from build123d import *

# Parameters (mm, degrees)
F0_R     = 11.45
F1_DEPTH = 7.62


# Not quite as in the source:
# - a feature names something its author has since deleted; it is built from what else it names


with BuildPart() as f1:
    # F0 (on Top) → F1 (new body)
    with BuildSketch(Plane.XY):
        with BuildLine():
            ThreePointArc((-10.038027058, 16.1907539288), (0, 19.05), (10.038027058, 16.1907539288))
            ThreePointArc((10.038027058, 16.1907539288), (8.1892299167, 26.451450684), (10.618228457, 36.59047997))
            ThreePointArc((10.618228457, 36.59047997), (0, 38.1), (-10.618228457, 36.59047997))
            ThreePointArc((-10.618228457, 36.59047997), (-8.1892299167, 26.451450684), (-10.038027058, 16.1907539288))
        make_face()
        with BuildLine():
            ThreePointArc((16.1907539288, -10.038027058), (18.3212494435, -5.2186510544), (19.05, 0))
            ThreePointArc((19.05, 0), (18.3212494435, 5.2186510544), (16.1907539288, 10.038027058))
            ThreePointArc((16.1907539288, 10.038027058), (15.2571196867, 11.4071380664), (14.208032523, 12.6899295438))
            ThreePointArc((14.208032523, 12.6899295438), (13.3304286547, 13.6089004655), (12.3935124609, 14.4673200311))
            ThreePointArc((12.3935124609, 14.4673200311), (11.2488242673, 15.3742138857), (10.038027058, 16.1907539288))
            ThreePointArc((10.038027058, 16.1907539288), (0, 19.05), (-10.038027058, 16.1907539288))
            ThreePointArc((-10.038027058, 16.1907539288), (-11.4071380664, 15.2571196867), (-12.6899295437, 14.208032523))
            ThreePointArc((-12.6899295437, 14.208032523), (-13.6089004655, 13.3304286548), (-14.467320031, 12.3935124609))
            ThreePointArc((-14.467320031, 12.3935124609), (-15.3742138857, 11.2488242673), (-16.1907539288, 10.038027058))
            ThreePointArc((-16.1907539288, 10.038027058), (-19.05, 0), (-16.1907539288, -10.038027058))
            ThreePointArc((-16.1907539288, -10.038027058), (-15.2571196867, -11.4071380664), (-14.208032523, -12.6899295437))
            ThreePointArc((-14.208032523, -12.6899295437), (-13.3304286548, -13.6089004655), (-12.3935124609, -14.467320031))
            ThreePointArc((-12.3935124609, -14.467320031), (-11.2488242673, -15.3742138857), (-10.038027058, -16.1907539288))
            ThreePointArc((-10.038027058, -16.1907539288), (0, -19.05), (10.038027058, -16.1907539288))
            ThreePointArc((10.038027058, -16.1907539288), (11.4071380664, -15.2571196867), (12.6899295438, -14.208032523))
            ThreePointArc((12.6899295438, -14.208032523), (13.6089004655, -13.3304286547), (14.4673200311, -12.3935124609))
            ThreePointArc((14.4673200311, -12.3935124609), (15.3742138857, -11.2488242673), (16.1907539288, -10.038027058))
        make_face()
        Circle(F0_R, mode=Mode.SUBTRACT)
        with BuildLine():
            ThreePointArc((-10.618228457, 36.59047997), (0, 38.1), (10.618228457, 36.59047997))
            ThreePointArc((10.618228457, 36.59047997), (10.9631553547, 37.2915593412), (11.3294826074, 37.9816978733))
            ThreePointArc((11.3294826074, 37.9816978733), (9.6714472488, 40.5242467677), (7.4026469551, 42.5407242305))
            ThreePointArc((7.4026469551, 42.5407242305), (0, 43.18), (-7.4026469551, 42.5407242305))
            ThreePointArc((-7.4026469551, 42.5407242305), (-9.6714472488, 40.5242467677), (-11.3294826074, 37.9816978733))
            ThreePointArc((-11.3294826074, 37.9816978733), (-10.9631553547, 37.2915593412), (-10.618228457, 36.59047997))
        make_face()
        with BuildLine():
            ThreePointArc((-27.6564265836, 26.2055732359), (-19.8292429656, 32.5332310632), (-10.618228457, 36.59047997))
            ThreePointArc((-10.618228457, 36.59047997), (-10.9631553547, 37.2915593412), (-11.3294826074, 37.9816978733))
            ThreePointArc((-11.3294826074, 37.9816978733), (-9.6714472488, 40.5242467677), (-7.4026469551, 42.5407242305))
            ThreePointArc((-7.4026469551, 42.5407242305), (-30.5262465043, 30.5394936821), (-42.5375084691, 7.4211032363))
            ThreePointArc((-42.5375084691, 7.4211032363), (-42.4698240182, 7.5132687267), (-42.401220917, 7.6047524795))
            ThreePointArc((-42.401220917, 7.6047524795), (-40.430781391, 9.7510814924), (-37.9816978733, 11.3294826074))
            ThreePointArc((-37.9816978733, 11.3294826074), (-37.2915593412, 10.9631553547), (-36.59047997, 10.618228457))
            ThreePointArc((-36.59047997, 10.618228457), (-33.6685368778, 17.8336654815), (-29.3410352271, 24.3046014533))
            ThreePointArc((-29.3410352271, 24.3046014533), (-28.5145767397, 25.2691296517), (-27.6564265836, 26.2055732359))
        make_face()
        with BuildLine():
            ThreePointArc((-11.3294826074, -37.9816978733), (-10.9631553547, -37.2915593412), (-10.618228457, -36.59047997))
            ThreePointArc((-10.618228457, -36.59047997), (-17.8336654815, -33.6685368778), (-24.3046014533, -29.3410352271))
            ThreePointArc((-24.3046014533, -29.3410352271), (-25.2691296517, -28.5145767397), (-26.2055732359, -27.6564265836))
            ThreePointArc((-26.2055732359, -27.6564265836), (-32.5332310632, -19.8292429656), (-36.59047997, -10.618228457))
            ThreePointArc((-36.59047997, -10.618228457), (-37.2915593412, -10.9631553547), (-37.9816978733, -11.3294826074))
            ThreePointArc((-37.9816978733, -11.3294826074), (-40.5242467677, -9.6714472488), (-42.5407242305, -7.4026469551))
            ThreePointArc((-42.5407242305, -7.4026469551), (-30.5328708116, -30.5328708116), (-7.4026469551, -42.5407242305))
            ThreePointArc((-7.4026469551, -42.5407242305), (-9.6714472488, -40.5242467677), (-11.3294826074, -37.9816978733))
        make_face()
        with BuildLine():
            Line((-24.3046014533, -29.3410352271), (-12.3935124609, -14.467320031))
            ThreePointArc((-12.3935124609, -14.467320031), (-13.3304286548, -13.6089004655), (-14.208032523, -12.6899295437))
            Line((-14.208032523, -12.6899295437), (-26.2055732359, -27.6564265836))
            ThreePointArc((-26.2055732359, -27.6564265836), (-25.2691296517, -28.5145767397), (-24.3046014533, -29.3410352271))
        make_face()
        with BuildLine():
            ThreePointArc((10.6182284569, -36.59047997), (8.1892299167, -26.451450684), (10.038027058, -16.1907539288))
            ThreePointArc((10.038027058, -16.1907539288), (0, -19.05), (-10.038027058, -16.1907539288))
            ThreePointArc((-10.038027058, -16.1907539288), (-8.1892299167, -26.451450684), (-10.618228457, -36.59047997))
            ThreePointArc((-10.618228457, -36.59047997), (0, -38.1), (10.6182284569, -36.59047997))
        make_face()
        with BuildLine():
            ThreePointArc((11.3294826074, -37.9816978733), (10.9631553547, -37.2915593412), (10.6182284569, -36.59047997))
            ThreePointArc((10.6182284569, -36.59047997), (0, -38.1), (-10.618228457, -36.59047997))
            ThreePointArc((-10.618228457, -36.59047997), (-10.9631553547, -37.2915593412), (-11.3294826074, -37.9816978733))
            ThreePointArc((-11.3294826074, -37.9816978733), (-9.6714472488, -40.5242467677), (-7.4026469551, -42.5407242305))
            ThreePointArc((-7.4026469551, -42.5407242305), (0, -43.18), (7.4026469551, -42.5407242305))
            ThreePointArc((7.4026469551, -42.5407242305), (9.6714472488, -40.5242467677), (11.3294826074, -37.9816978733))
        make_face()
        with BuildLine():
            ThreePointArc((37.9816978733, 11.3294826074), (37.2915593412, 10.9631553547), (36.59047997, 10.6182284569))
            ThreePointArc((36.59047997, 10.6182284569), (37.7207322759, 5.3624953679), (38.1, 0))
            ThreePointArc((38.1, 0), (37.7207322759, -5.3624953679), (36.59047997, -10.618228457))
            ThreePointArc((36.59047997, -10.618228457), (37.2915593412, -10.9631553547), (37.9816978733, -11.3294826074))
            ThreePointArc((37.9816978733, -11.3294826074), (40.5242467677, -9.6714472488), (42.5407242305, -7.4026469551))
            ThreePointArc((42.5407242305, -7.4026469551), (43.0198841948, -3.7150994419), (43.18, 0))
            ThreePointArc((43.18, 0), (43.0198841948, 3.7150994419), (42.5407242305, 7.4026469551))
            ThreePointArc((42.5407242305, 7.4026469551), (40.5242467677, 9.6714472488), (37.9816978733, 11.3294826074))
        make_face()
        with BuildLine():
            ThreePointArc((16.1907539288, 10.038027058), (18.3212494435, 5.2186510544), (19.05, 0))
            ThreePointArc((19.05, 0), (18.3212494435, -5.2186510544), (16.1907539288, -10.038027058))
            ThreePointArc((16.1907539288, -10.038027058), (26.451450684, -8.1892299167), (36.59047997, -10.618228457))
            ThreePointArc((36.59047997, -10.618228457), (37.7207322759, -5.3624953679), (38.1, 0))
            ThreePointArc((38.1, 0), (37.7207322759, 5.3624953679), (36.59047997, 10.6182284569))
            ThreePointArc((36.59047997, 10.6182284569), (26.451450684, 8.1892299167), (16.1907539288, 10.038027058))
        make_face()
        with BuildLine():
            Line((29.3410352271, -24.3046014533), (14.467320031, -12.3935124609))
            ThreePointArc((14.4673200311, -12.3935124609), (13.6089004655, -13.3304286547), (12.6899295438, -14.208032523))
            Line((12.6899295437, -14.208032523), (27.6564265836, -26.2055732359))
            ThreePointArc((27.6564265836, -26.2055732359), (28.5145767397, -25.2691296517), (29.3410352271, -24.3046014533))
        make_face()
        with BuildLine():
            ThreePointArc((-14.467320031, 12.3935124609), (-13.6089004655, 13.3304286548), (-12.6899295437, 14.208032523))
            Line((-12.6899295437, 14.208032523), (-27.6564265836, 26.2055732359))
            ThreePointArc((-27.6564265836, 26.2055732359), (-28.5145767397, 25.2691296517), (-29.3410352271, 24.3046014533))
            Line((-29.3410352271, 24.3046014533), (-14.467320031, 12.3935124609))
        make_face()
        with BuildLine():
            ThreePointArc((12.3935124609, 14.4673200311), (13.3304286547, 13.6089004655), (14.208032523, 12.6899295438))
            Line((14.208032523, 12.6899295438), (26.2055732359, 27.6564265836))
            ThreePointArc((26.2055732359, 27.6564265836), (25.2691296517, 28.5145767397), (24.3046014533, 29.3410352271))
            Line((24.3046014533, 29.3410352271), (12.3935124609, 14.4673200311))
        make_face()
        with BuildLine():
            ThreePointArc((37.9816978733, -11.3294826074), (37.2915593412, -10.9631553547), (36.59047997, -10.618228457))
            ThreePointArc((36.59047997, -10.618228457), (33.6685368778, -17.8336654815), (29.3410352271, -24.3046014533))
            ThreePointArc((29.3410352271, -24.3046014533), (28.5145767397, -25.2691296517), (27.6564265836, -26.2055732359))
            ThreePointArc((27.6564265836, -26.2055732359), (19.8292429656, -32.5332310632), (10.6182284569, -36.59047997))
            ThreePointArc((10.6182284569, -36.59047997), (10.9631553547, -37.2915593412), (11.3294826074, -37.9816978733))
            ThreePointArc((11.3294826074, -37.9816978733), (9.6714472488, -40.5242467677), (7.4026469551, -42.5407242305))
            ThreePointArc((7.4026469551, -42.5407242305), (30.5328708116, -30.5328708116), (42.5407242305, -7.4026469551))
            ThreePointArc((42.5407242305, -7.4026469551), (40.5242467677, -9.6714472488), (37.9816978733, -11.3294826074))
        make_face()
        with BuildLine():
            ThreePointArc((26.2055732359, 27.6564265836), (32.5332310632, 19.8292429656), (36.59047997, 10.6182284569))
            ThreePointArc((36.59047997, 10.6182284569), (37.2915593412, 10.9631553547), (37.9816978733, 11.3294826074))
            ThreePointArc((37.9816978733, 11.3294826074), (40.5242467677, 9.6714472488), (42.5407242305, 7.4026469551))
            ThreePointArc((42.5407242305, 7.4026469551), (30.5328708116, 30.5328708116), (7.4026469551, 42.5407242305))
            ThreePointArc((7.4026469551, 42.5407242305), (9.6714472488, 40.5242467677), (11.3294826074, 37.9816978733))
            ThreePointArc((11.3294826074, 37.9816978733), (10.9631553547, 37.2915593412), (10.618228457, 36.59047997))
            ThreePointArc((10.618228457, 36.59047997), (17.8336654815, 33.6685368778), (24.3046014533, 29.3410352271))
            ThreePointArc((24.3046014533, 29.3410352271), (25.2691296517, 28.5145767397), (26.2055732359, 27.6564265836))
        make_face()
        with BuildLine():
            ThreePointArc((-16.1907539288, -10.038027058), (-19.05, 0), (-16.1907539288, 10.038027058))
            ThreePointArc((-16.1907539288, 10.038027058), (-26.451450684, 8.1892299167), (-36.59047997, 10.618228457))
            ThreePointArc((-36.59047997, 10.618228457), (-38.1, 0), (-36.59047997, -10.618228457))
            ThreePointArc((-36.59047997, -10.618228457), (-26.451450684, -8.1892299167), (-16.1907539288, -10.038027058))
        make_face()
        with BuildLine():
            ThreePointArc((-42.5407242305, 7.4026469551), (-43.18, 0), (-42.5407242305, -7.4026469551))
            ThreePointArc((-42.5407242305, -7.4026469551), (-40.5242467677, -9.6714472488), (-37.9816978733, -11.3294826074))
            ThreePointArc((-37.9816978733, -11.3294826074), (-37.2915593412, -10.9631553547), (-36.59047997, -10.618228457))
            ThreePointArc((-36.59047997, -10.618228457), (-38.1, 0), (-36.59047997, 10.618228457))
            ThreePointArc((-36.59047997, 10.618228457), (-37.2915593412, 10.9631553547), (-37.9816978733, 11.3294826074))
            ThreePointArc((-37.9816978733, 11.3294826074), (-40.430781391, 9.7510814924), (-42.401220917, 7.6047524795))
            ThreePointArc((-42.401220917, 7.6047524795), (-42.4715153756, 7.5040743862), (-42.5407242305, 7.4026469551))
        make_face()
    extrude(amount=F1_DEPTH)


solid = f1.part
The listing builds one solid part. Answer for the finished solid, in the listing's coordinates (mm). A direction names the side the tool comes from. Coordinates: 2 decimals unless noted, no trailing zeros. Order: outer loops, then holes, each group sorted by start corner. A loop starts at its lowest first (then second) coordinate and runs counter-clockwise, first axis right, second up. Notation, with made-up numbers: (64.5, 42) -> (84.5, 42) arc R25 ccw to (84.5, 64) -> close; hole circle Ø6 at (-7, 27). An arc over 180 degrees is marked (long way). Answer in a Markdown table with one row per item. Add a question column.
Item 1: Determine the mould class of faces 3 (the face through (-26.598, -8.194, 3.757)), 4 (the face through (9, -9, 0)), 5 (the face through (19.95, -32.46, 3.76)) for opening direction Y: +Y half, -Y half, draft (parallel to the pull), parting line (faces both ways), or undercut.
Item 2: Find the intervals of material crossed by L1, parallel to Y at x = -22, z = 3.75; L2, parallel to X at y = -24, z = 3.5; L3, parallel to Y at x = -23, z = 2.5, in increasing order. Write a range as from..to.
Item 3: Find section B-B (y = 33). Write down the section's boundary in (x, z).
Item 4: Each of these flat-tipped pins is pushed along its axis until it touches: P1, Ø1.5, axis at y = 33.5, z = 4.5, coming from the -X side; P2, Ø1.5, axis at x = 20, y = 5, coming from the -Z side; P3, Ø18.5, axis at x = 0, y = 0, coming from the +Z side; P4, Ø1.5, axis at y = -26, z = 2.5, coming from the +X side. Where does it stop, or does it pass through?
Item 5: Find section C-C (x = 17.5). Write down the section's boundary in (y, z), then the cut area to 3 significant figures.
Item 6: Find section A-A (x = 0). Write down the section's boundary in (y, z).
Item 7: Which of the six approach directions +Z, -Z, +X, -X, +Y, -Y give full straight-line access (tool end or side, diameter ignored) to faces 1 (the face through (33.72, -17.74, 3.76)), 2 (the face through (9, -9, 7.62))?
Item 8: Find section D-D (x = 32). Write down the section's boundary in (y, z).
Result set:
| question | item | result |
|---|---|---|
| 1 | face 3 | undercut |
| 1 | face 4 | draft |
| 1 | face 5 | undercut |
| 2 | L1 | y = -37.16..-31.11, -26.46..-22.41, -8.45..8.45, 18.43..21.67, 31.11..37.16 |
| 2 | L2 | x = -35.9..-29.59, -23.27..-20.03, -8.24..8.24, 24.91..28.96, 29.59..35.9 |
| 2 | L3 | y = -36.54..-30.37, -27.71..-23.66, -8.33..8.33, 19.23..22.47, 30.37..36.54 |
| 3 | outline | (-27.85, 0) -> (-19.04, 0) -> (-19.04, 7.62) -> (-27.85, 7.62) -> close; (-9.24, 0) -> (9.24, 0) -> (9.24, 7.62) -> (-9.24, 7.62) -> close; (19.04, 0) -> (27.85, 0) -> (27.85, 7.62) -> (19.04, 7.62) -> close |
| 4 | P1 | stops at x = -28.14 |
| 4 | P2 | stops at z = 0 |
| 4 | P3 | passes through |
| 4 | P4 | stops at x = 35.03 |
| 5 | outline | (-39.47, 0) -> (-33.84, 0) -> (-33.84, 7.62) -> (-39.47, 7.62) -> close; (-18.06, 0) -> (-14.82, 0) -> (-14.82, 7.62) -> (-18.06, 7.62) -> close; (-9.55, 0) -> (9.55, 0) -> (9.55, 7.62) -> (-9.55, 7.62) -> close; (16.8, 0) -> (20.84, 0) -> (20.84, 7.62) -> (16.8, 7.62) -> close; (33.84, 0) -> (39.47, 0) -> (39.47, 7.62) -> (33.84, 7.62) -> close |
| 5 | area | 287 mm² |
| 6 | outline | (-43.18, 0) -> (-11.45, 0) -> (-11.45, 7.62) -> (-43.18, 7.62) -> close; (11.45, 0) -> (43.18, 0) -> (43.18, 7.62) -> (11.45, 7.62) -> close |
| 7 | face 1 | +Z, -Z |
| 7 | face 2 | +Z, +X, -X, +Y, -Y |
| 8 | outline | (-28.99, 0) -> (-20.68, 0) -> (-20.68, 7.62) -> (-28.99, 7.62) -> close; (-8.97, 0) -> (8.97, 0) -> (8.97, 7.62) -> (-8.97, 7.62) -> close; (20.68, 0) -> (28.99, 0) -> (28.99, 7.62) -> (20.68, 7.62) -> close |
